from build123d import *

# Parameters (mm, degrees)
ESQUISSE1_W             = 40.8
ESQUISSE1_H             = 20
BOSS_EXTRU_1_DEPTH      = 35.3
BOSS_EXTRU_2_DEPTH      = 2
ESQUISSE3_R             = 6.4
BOSS_EXTRU_3_DEPTH      = 1.5
ESQUISSE4_R             = 2.9
ESQUISSE4_R_2           = 1.3
BOSS_EXTRU_4_DEPTH      = 4
ESQUISSE5_W             = 7
ESQUISSE5_H             = 20
BOSS_EXTRU_5_DEPTH      = 2
ENL_V_MAT_EXTRU_1_DEPTH = 59.428075443
CONG_1_R                = 2
ESQUISSE7_W             = 4
ESQUISSE7_H             = 7
BOSS_EXTRU_6_DEPTH      = 10
CHANFREIN1_SIZE         = 2
CONG_2_R                = 1


with BuildPart() as part:
    # Esquisse1 → Boss.-Extru.1 (new body)
    with BuildSketch(Plane.XY):
        with Locations((20.4, 10)):
            Rectangle(ESQUISSE1_W, ESQUISSE1_H)
    extrude(amount=BOSS_EXTRU_1_DEPTH)

    # Esquisse2 → Boss.-Extru.2 (add)
    with BuildSketch(Plane.XY.offset(35.3)):
        with BuildLine():
            Line((14.358898944, 19), (34.8, 19))
            Line((34.8, 19), (34.8, 15))
            ThreePointArc((34.8, 15), (39.8, 10), (34.8, 5))
            Line((34.8, 5), (34.8, 1))
            Line((34.8, 1), (14.358898944, 1))
            ThreePointArc((14.358898944, 1), (0, 10), (14.358898944, 19))
        make_face()
    extrude(amount=BOSS_EXTRU_2_DEPTH)

    # Esquisse3 → Boss.-Extru.3 (add)
    with BuildSketch(Plane.XY.offset(37.3)):
        with Locations((10, 10)):
            Circle(ESQUISSE3_R)
    extrude(amount=BOSS_EXTRU_3_DEPTH)

    # Esquisse4 → Boss.-Extru.4 (add)
    with BuildSketch(Plane.XY.offset(38.8)):
        with Locations((10, 10)):
            Circle(ESQUISSE4_R)
        with Locations((10, 10)):
            Circle(ESQUISSE4_R_2, mode=Mode.SUBTRACT)
    extrude(amount=BOSS_EXTRU_4_DEPTH)

    # Esquisse5 → Boss.-Extru.5 (add)
    with BuildSketch(Plane(origin=(0, 0, 27), x_dir=(-1, 0, 0), z_dir=(0, 0, -1))):
        with Locations((-44.3, 10)):
            Rectangle(ESQUISSE5_W, ESQUISSE5_H)
        with Locations((3.5, 10)):
            Rectangle(ESQUISSE5_W, ESQUISSE5_H)
    extrude(amount=BOSS_EXTRU_5_DEPTH)

    # Esquisse6 → Enlèv. mat.-Extru.1 (cut, through all)
    with BuildSketch(Plane.XY.offset(27)):
        with BuildLine():
            Line((-6.721320344, 15.75), (-7, 15.75))
            Line((-7, 15.75), (-7, 14.25))
            Line((-7, 14.25), (-6.721320344, 14.25))
            ThreePointArc((-6.721320344, 14.25), (-2.35, 15), (-6.721320344, 15.75))
        make_face()
        with BuildLine():
            Line((47.521320344, 14.25), (47.8, 14.25))
            Line((47.8, 14.25), (47.8, 15.75))
            Line((47.8, 15.75), (47.521320344, 15.75))
            ThreePointArc((47.521320344, 15.75), (43.15, 15), (47.521320344, 14.25))
        make_face()
        with BuildLine():
            Line((47.521320344, 4.25), (47.8, 4.25))
            Line((47.8, 4.25), (47.8, 5.75))
            Line((47.8, 5.75), (47.521320344, 5.75))
            ThreePointArc((47.521320344, 5.75), (43.15, 5), (47.521320344, 4.25))
        make_face()
        with BuildLine():
            Line((-6.721320344, 5.75), (-7, 5.75))
            Line((-7, 5.75), (-7, 4.25))
            Line((-7, 4.25), (-6.721320344, 4.25))
            ThreePointArc((-6.721320344, 4.25), (-2.35, 5), (-6.721320344, 5.75))
        make_face()
    extrude(amount=-ENL_V_MAT_EXTRU_1_DEPTH, mode=Mode.SUBTRACT)

    # Congé1
    cong_1_edges = [part.edges().sort_by_distance(p)[0] for p in [
        (47.8, 20, 26),
        (47.8, 0, 26),
        (-7, 20, 26),
        (-7, 0, 26),
    ]]
    fillet(cong_1_edges, radius=CONG_1_R)

    # Esquisse7 → Boss.-Extru.6 (add)
    with BuildSketch(Plane.ZY):
        with Locations((5, 10)):
            Rectangle(ESQUISSE7_W, ESQUISSE7_H)
    extrude(amount=BOSS_EXTRU_6_DEPTH)

    # Chanfrein1
    chanfrein1_edges = [part.edges().sort_by_distance(p)[0] for p in [
        (20.4, 20, 0),
        (40.8, 10, 0),
        (20.4, 0, 0),
        (0, 10, 0),
    ]]
    chamfer(chanfrein1_edges, length=CHANFREIN1_SIZE)

    # Congé2
    cong_2_edges = [part.edges().sort_by_distance(p)[0] for p in [
        (-5, 6.5, 7),
        (-5, 13.5, 7),
        (-5, 13.5, 3),
        (-5, 6.5, 3),
    ]]
    fillet(cong_2_edges, radius=CONG_2_R)


solid = part.part
Geometry: final body of the model. Coordinates: model frame, mm. A direction names the side the tool comes from. Give positions to 0.01 mm unless a question says otherwise; leave off trailing zeros. Write each loop counter-clockwise with the first axis right and the second up, starting at its lowest first coordinate (ties: lowest second). Pieces come first, ordered by that corner, then holes. Notation, with made-up numbers: (17, 57.25) -> (42, 57.25) arc R17 ccw to (42, 75.25) -> close; hole circle Ø2 at (66, 7.5). An arc over 180 degrees is marked (long way). Answer as a JSON object with one key per item and string values.
1. Cut plane A-A on z = 36.5. Output: boundary loops of the cut face in (x, y).
Ans:
{"outline": "(14.36, 1) -> (34.8, 1) -> (34.8, 5) arc R5 ccw to (34.8, 15) -> (34.8, 19) -> (14.36, 19) arc R10 ccw (long way) to start"}
2. Contact query for flat-ended pins moving along their axis: pin 1 (3 mm diameter, centred on x = -1, z = 22, fed in from +Y); pin 2 (6 mm diameter, centred on y = 9.5, z = 32.5, fed in from -X); pin 3 (0.6 mm diameter, centred on x = -7.5, z = 5, fed in from -Y); pin 4 (3.5 mm diameter, centred on x = -4.6, y = 5, fed in from +Z). Output: stop coordinate, or through.
Ans:
{"pin 1": "stops at y = 20", "pin 2": "stops at x = 0", "pin 3": "stops at y = 6.5", "pin 4": "stops at z = 6.66"}
3. Mould query, pull axis Y, two halves, no side actions, for faces 6 (the flat face through (44, 10, 25)), 7 (the cylindrical face through (43.15, 15.09, 26.01)), 8 (the cylindrical face through (0, 10, 36)), 9 (the cylindrical face through (-2.35, 14.91, 26.01)). Classes: pulls with the +Y half, pulls with the -Y half, needs draft (parallel to the pull), parting line crosses it, or undercut.
Ans:
{"face 6": "needs draft", "face 7": "undercut", "face 8": "parting line crosses it", "face 9": "undercut"}
4. Cut plane B-B on x = -3.5. Output: boundary loops of the cut face in (y, z), and give its area (3 significant figures).
Ans:
{"outline": "(0, 25) -> (3.04, 25) -> (3.04, 27) -> (0, 27) -> close; (6.5, 4) arc R1 ccw to (7.5, 3) -> (12.5, 3) arc R1 ccw to (13.5, 4) -> (13.5, 6) arc R1 ccw to (12.5, 7) -> (7.5, 7) arc R1 ccw to (6.5, 6) -> close; (6.96, 25) -> (13.04, 25) -> (13.04, 27) -> (6.96, 27) -> close; (16.96, 25) -> (20, 25) -> (20, 27) -> (16.96, 27) -> close", "area": "51.4 mm^2"}
5. Cut plane D-D on z = 5. Output: boundary loops of the cut face in (x, y).
Ans:
{"outline": "(-10, 6.5) -> (0, 6.5) -> (0, 0) -> (40.8, 0) -> (40.8, 20) -> (0, 20) -> (0, 13.5) -> (-10, 13.5) -> close"}
6. Access query for faces 1 (the flat face through (-7, 10, 26)), 2 (the flat face through (34.8, 3, 36)), 3 (the flat face through (-5, 10, 7)), 4 (the cylindrical face through (7.1, 10.1, 40.8)), 5 (the flat face through (-5, 6.5, 5)). Directions: +Z, -Z, +X, -X, +Y, -Y. A direction counts if a zero-diameter tool reaches every point of the face in a straight line with its end or side. Return the directions, or none.
Ans:
{"face 1": "+Z, -X, +Y, -Y", "face 2": "+Z, +X, -Y", "face 3": "-X, +Y, -Y", "face 4": "+Z", "face 5": "-Z, -X, -Y"}
7. Ray query, probe 1 along Y at (x, z) = (45.4, 26.55); probe 2 along X at (y, z) = (12.75, 33); probe 3 along Z at (x, y) = (34, 2.75). Return the intervals inside material, ascending. Write a range as from..to.
Ans:
{"probe 1": "y = 0..2.75, 7.25..12.75, 17.25..20", "probe 2": "x = 0..40.8", "probe 3": "z = 0..37.3"}
8. Cut plane C-C on x = 22. Output: boundary loops of the cut face in (y, z).
Ans:
{"outline": "(0, 2) -> (2, 0) -> (18, 0) -> (20, 2) -> (20, 35.3) -> (19, 35.3) -> (19, 37.3) -> (1, 37.3) -> (1, 35.3) -> (0, 35.3) -> close"}
